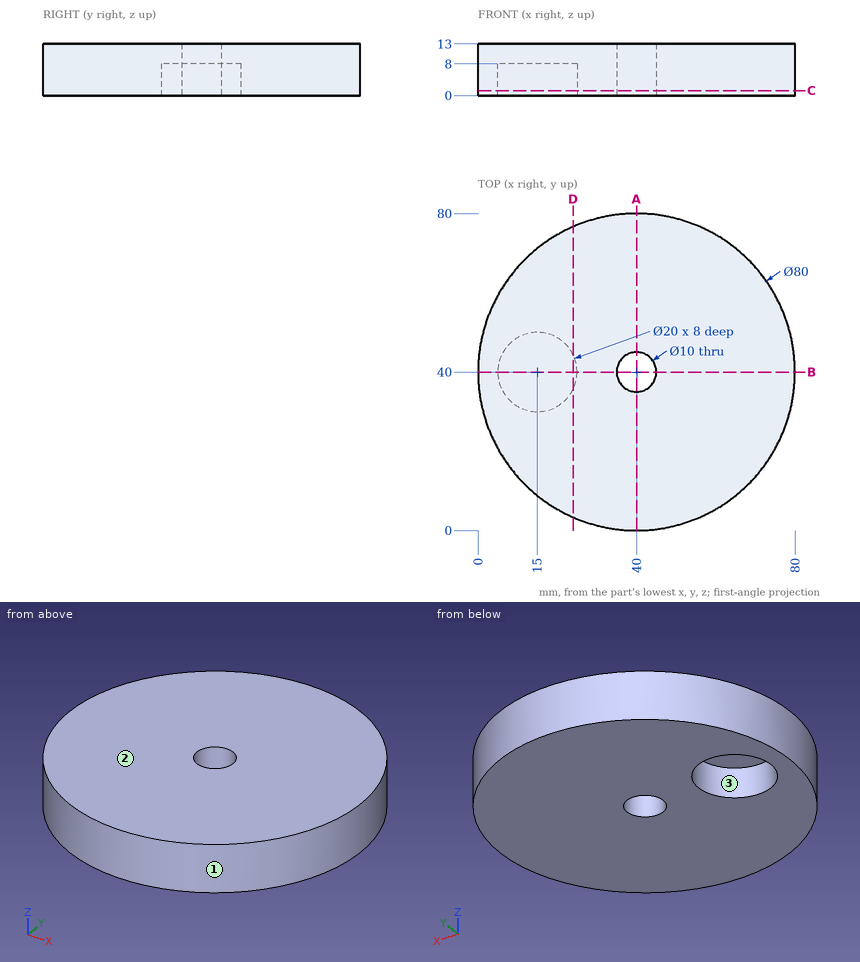
Could you check a few things on this drawing? It's one solid part, dimensions in mm from its lowest x, y, z. Round coordinates to 2 decimals unless told otherwise and drop trailing zeros. Loops run counter-clockwise (first coordinate to the right, second up) from the corner with the lowest first, then second, coordinate; pieces in that order, holes last.
Q1. I want a section at B-B (y = 40). Write out the boundary of the cut face in (x, z).
Q2. I want a section at A-A (x = 40). Write out the boundary of the cut face in (y, z), and give its area (3 significant figures).
Q3. I want a section at C-C (z = 1.25). Write out the boundary of the cut face in (x, y).
Q4. For P1, Ø3, axis at x = 28, z = 4.5, coming from the -Y side; P2, Ø4, axis at x = 11, z = 6, coming from the +Y side; P3, Ø4, axis at x = 71.5, z = 8, coming from the +Y side, each with a flat end and sliding along its axis, tell me the tip position at first contact or that it passes through.
Q5. Thinking about a two-plate mould opening in Y: for the marked faces 1, 2 and 3, which applies, pulls with the +Y half, pulls with the -Y half, needs draft (parallel to the pull), parting line crosses it, or undercut?
Q6. I want a section at D-D (x = 24). Write out the boundary of the cut face in (y, z).
Q7. Please list where these lines run through material, in increasing order: L1, parallel to Y at x = 40, z = 4.5; L2, parallel to Z at x = 13, y = 39.5; L3, parallel to Y at x = 15, z = 2.
Answer below:
1. outline: (0, 0) - (5, 0) - (5, 8) - (25, 8) - (25, 0) - (35, 0) - (35, 13) - (0, 13) - close; (45, 0) - (80, 0) - (80, 13) - (45, 13) - close
2. outline: (0, 0) - (35, 0) - (35, 13) - (0, 13) - close; (45, 0) - (80, 0) - (80, 13) - (45, 13) - close
2. area: 910 mm2
3. outline: circle Ø80 at (40, 40); hole circle Ø20 at (15, 40); hole circle Ø10 at (40, 40)
4. P1: stops at y = 1.4
4. P2: stops at y = 69.51
4. P3: stops at y = 67.01
5. face 1: parting line crosses it
5. face 2: needs draft
5. face 3: undercut
6. outline: (3.34, 0) - (35.64, 0) - (35.64, 8) - (44.36, 8) - (44.36, 0) - (76.66, 0) - (76.66, 13) - (3.34, 13) - close
7. L1: y = 0 to 35, 45 to 80
7. L2: z = 8 to 13
7. L3: y = 8.78 to 30, 50 to 71.22
